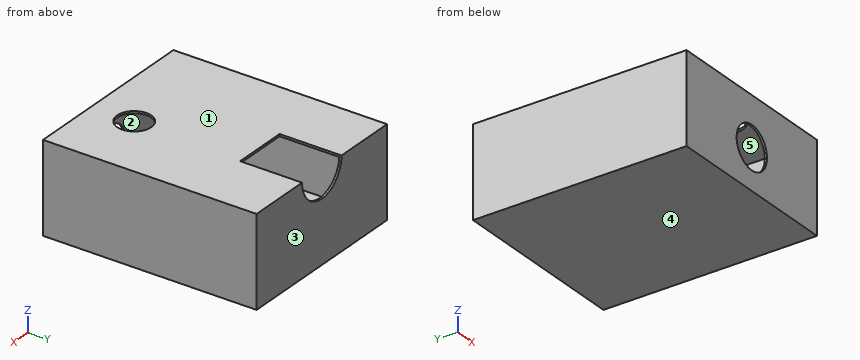
from build123d import *

# Parameters (mm, degrees)
F1_DEPTH = 500
F2_T     = -5
F4_DEPTH = 5
F5_DEPTH = 10
F6_W     = 130.1
F6_H     = 350
F7_DEPTH = 5
F8_R     = 40
F9_DEPTH = 25


# Not quite as in the source:
# - a feature names something its author has since deleted; it is built from what else it names


with BuildPart() as f1:
    # F0 (on Front) → F1 (new body)
    with BuildSketch(Plane.XZ):
        with BuildLine():
            Line((-133.7995099491, 37.318477902), (-133.7995099491, -172.681522098))
            Line((-133.7995099491, -172.681522098), (296.3004900509, -172.681522098))
            Line((296.3004900509, -172.681522098), (296.3004900509, 37.318477902))
            Line((296.3004900509, 37.318477902), (146.3004900509, 37.318477902))
            ThreePointArc((146.3004900509, 37.318477902), (81.2504900509, -27.731522098), (16.2004900509, 37.318477902))
            Line((16.2004900509, 37.318477902), (-133.7995099491, 37.318477902))
        make_face()
    extrude(amount=F1_DEPTH)

    # F2
    f2_openings = [f1.faces().sort_by_distance(p)[0] for p in [
        (81.25049, -250, -27.731522),
    ]]
    offset(amount=F2_T, openings=f2_openings)

    # F3 (on face) → F4 (join)
    with BuildSketch(Plane.XZ.offset(500)):
        with BuildLine():
            Line((146.3004900509, 37.318477902), (16.2004900509, 37.318477902))
            ThreePointArc((16.2004900509, 37.318477902), (35.2531939347, -8.6788182142), (81.2504900509, -27.731522098))
            ThreePointArc((81.2504900509, -27.731522098), (127.2477861671, -8.6788182142), (146.3004900509, 37.318477902))
        make_face()
    extrude(amount=-F4_DEPTH)

    # F3 (on face) → F5 (cut)
    with BuildSketch(Plane.XZ.offset(500)):
        with BuildLine():
            ThreePointArc((81.2504900509, -27.731522098), (45.8951509916, -113.0868611574), (131.2504900509, -77.731522098))
            ThreePointArc((131.2504900509, -77.731522098), (116.6058291102, -42.3761830387), (81.2504900509, -27.731522098))
        make_face()
    extrude(amount=-F5_DEPTH, mode=Mode.SUBTRACT)

    # F6 (on face) → F7 (join)
    with BuildSketch(Plane.XY.offset(37.318477902)):
        with Locations((81.2504900509, -320)):
            Rectangle(F6_W, F6_H)
    extrude(amount=-F7_DEPTH)

    # F8 (on face) → F9 (cut)
    with BuildSketch(Plane.XY.offset(37.318477902)):
        with Locations((136.3004900509, -400)):
            Circle(F8_R)
    extrude(amount=-F9_DEPTH, mode=Mode.SUBTRACT)


solid = f1.part
CAD build for the part. Positions are in the model's coordinates, mm. Face numbers are marked on the shaded views. A direction names the side the tool comes from. Round coordinates to 2 decimals unless told otherwise and drop trailing zeros. Loops run counter-clockwise (first coordinate to the right, second up) from the corner with the lowest first, then second, coordinate; pieces in that order, holes last. Notation, with made-up numbers: M 32.25,65.25 L 55.25,65.25 A15 ccw 55.25,93.25 Z; hole C 28.5,-16 d11. An arc over 180 degrees is marked long. One line per question, with ' | ' between items. Start each with the question number.
Item 1: Two-plate mould, pull along Z, no slides. Class the marked faces 1, 2 and 3: pulls with the +Z half, pulls with the -Z half, needs draft (parallel to the pull), parting line crosses it, or undercut.
Item 2: Cut at A-A, the plane x = 43.5. Write the cut outline in (y, z).
Item 3: Wall check: line 1 (X direction, y = -437.5, z = -31); line 2 (Z direction, x = 101.5, y = -349.5); line 3 (Y direction, x = -7, z = 18.5). Give the ranges that are in metal, low to high.
Item 4: Which spindle directions (+Z, -Z, +X, -X, +Y, -Y) get a long thin tool onto all of the face, cutting with end or side? Do the marked faces 4 and 5. Say none if no direction does.
Item 5: Cut at D-D, the plane y = -461. Write the cut outline in (x, z), plus the area to 3 significant figures.
Item 6: Cut at C-C, the plane z = -147. Write the cut outline in (x, y), plus the area to 3 significant figures.
Item 7: Cut at B-B, the plane y = -400. Write the cut outline in (x, z).
Item 8: Pin check, flat tip, straight feed: pin 1 Ø4 at (x, z) = (77, 34) entering from +Y. Stop position of the tip, or through.
Responses:
1) face 1: pulls with the +Z half | face 2: undercut | face 3: needs draft
2) outline: M -500,-172.68 L 0,-172.68 L 0,-15.66 L -5,-15.66 L -5,-167.68 L -495,-167.68 L -495,-110.52 L -500,-110.52 Z; M -500,-44.95 L -495,-44.95 L -495,32.32 L -145,32.32 L -145,37.32 L -500,37.32 Z
3) line 1: x = -133.8 to -128.8, 291.3 to 296.3 | line 2: z = -172.68 to -167.68, 32.32 to 37.32 | line 3: y = -500 to -495, -5 to 0
4) face 4: -Z, +X, -X, +Y, -Y | face 5: none
5) outline: M -133.8,-172.68 L 296.3,-172.68 L 296.3,37.32 L -133.8,37.32 Z; hole M -128.8,-167.68 L 291.3,-167.68 L 291.3,32.32 L -128.8,32.32 Z | area: 6,300 mm²
6) outline: M -133.8,-500 L 296.3,-500 L 296.3,0 L -133.8,0 Z; hole M -128.8,-495 L 291.3,-495 L 291.3,-5 L -128.8,-5 Z | area: 9,200 mm²
7) outline: M -133.8,-172.68 L 296.3,-172.68 L 296.3,37.32 L 176.3,37.32 L 176.3,32.32 L 291.3,32.32 L 291.3,-167.68 L -128.8,-167.68 L -128.8,32.32 L 96.3,32.32 L 96.3,37.32 L -133.8,37.32 Z
8) pin 1: stops at y = -145
